Source: CAD feature listing. Evaluate the final solid. Frame: model axes, mm. A direction names the side the tool comes from. Round coordinates to 2 decimals unless told otherwise and drop trailing zeros.
```python
from build123d import *

# Parameters (mm, degrees)
F0_W      = 130.175
F0_H      = 33.3375
F1_DEPTH  = 11.1125
F2_R      = 8.73125
F2_R_2    = 4.7625
F3_DEPTH  = 6.35
F3_FACE_R = 4.7625
F4_DEPTH  = 11.1135
F5_R      = 1.5875
F6_DEPTH  = 6.35
F5_R_2    = 3.175
F7_DEPTH  = 11.1135
F5_R_3    = 4.7625
F8_DEPTH  = 6.35


with BuildPart() as f1:
    # F0 (on Top) → F1 (new body)
    with BuildSketch(Plane.XY):
        Rectangle(F0_W, F0_H)
    extrude(amount=F1_DEPTH)

    # F2 (on face) → F3 (cut)
    with BuildSketch(Plane.XY.offset(11.1125)):
        Circle(F2_R)
        Circle(F2_R_2, mode=Mode.SUBTRACT)
    extrude(amount=-F3_DEPTH, mode=Mode.SUBTRACT)

    # F3_face (on face) → F4 (cut, through all)
    with BuildSketch(Plane.XY.offset(11.1125)):
        Circle(F3_FACE_R)
    extrude(amount=-F4_DEPTH, mode=Mode.SUBTRACT)

    # F5 (on face) → F6 (cut)
    with BuildSketch(Plane.XY):
        with Locations((-49.2125, 0)):
            Circle(F5_R)
        with Locations((49.2125, 0)):
            Circle(F5_R)
    extrude(amount=F6_DEPTH, mode=Mode.SUBTRACT)

    # F5 (on face) → F7 (cut, through all)
    with BuildSketch(Plane.XY):
        with Locations((31.75, 0)):
            Circle(F5_R_2)
    extrude(amount=F7_DEPTH, mode=Mode.SUBTRACT)

    # F5 (on face) → F8 (cut)
    with BuildSketch(Plane.XY):
        with Locations((31.75, 0)):
            Circle(F5_R_3)
        with Locations((31.75, 0)):
            Circle(F5_R_2, mode=Mode.SUBTRACT)
    extrude(amount=F8_DEPTH, mode=Mode.SUBTRACT)


solid = f1.part
```
1. Line query: line 1 along Y through (x, z) = (31.75, 2.75); line 2 along Y through (x, z) = (31.75, 7.7) (3 decimals); line 3 along X through (y, z) = (5.5, 5). Output: solid intervals per line, ascending.
2. Pull-direction query (X, two-part tool) for faces 1 (the face through (-1, 11, 11.112)), 2 (the face through (65.088, 0, 5)), 3 (the face through (-49, 0, 6.35)); classes: released by +X, released by -X, zero draft, split by the parting line, or undercut.
3. First-contact query: pin 1 (5 mm diameter, centred on x = -3.5, y = -2.5, fed in from +Z); pin 2 (1 mm diameter, centred on x = 49, y = 0, fed in from -Z). Flat tips, straight axial feed; report the tip coordinate or a pass-through.
4. Section A-A on y = 0. State how many separate pieces and enclosed holes the cut face has, plus the area to 3 significant figures.
5. Access query for faces 4 (the face through (-6.93, -5.31, 7.98)), 5 (the face through (35, -1, 6.35)), 6 (the face through (28.58, 0.14, 8.7)). Directions: +Z, -Z, +X, -X, +Y, -Y. A direction counts if a zero-diameter tool reaches every point of the face in a straight line with its end or side. Return the directions, or none.
Result:
1. line 1: y = -16.67 to -4.76, 4.76 to 16.67
1. line 2: y = -16.669 to -3.175, 3.175 to 16.669
1. line 3: x = -65.09 to -6.78, 6.78 to 65.09
2. face 1: zero draft
2. face 2: released by +X
2. face 3: undercut
3. pin 1: stops at z = 4.76
3. pin 2: stops at z = 6.35
4. separate pieces: 3
4. enclosed holes: 0
4. area: 1,160 mm2
5. face 4: +Z
5. face 5: -Z
5. face 6: +Z, -Z
